The model under review builds one solid part; all positions refer to its coordinate system, in mm. A direction names the side the tool comes from. Round coordinates to 2 decimals unless told otherwise and drop trailing zeros. Loops run counter-clockwise (first coordinate to the right, second up) from the corner with the lowest first, then second, coordinate; pieces in that order, holes last. Notation, with made-up numbers: (31, 38) -> (65, 38) arc R31 ccw to (65, 70) -> close; hole circle Ø10 at (-33.75, -16.75). An arc over 180 degrees is marked (long way). Use a Markdown table: item, result. Add a question column.
1) For faces 4 (the cylindrical face through (1.449, 81.022, 3.219)), 5 (the flat face through (79.375, 41, 5)), list the 3-axis set-ups (+Z, -Z, +X, -X, +Y, -Y) from which the entire face can be reached by the end or side of a thin tool; tool diameter is ignored.
2) Mouldability with a two-part tool opening along X and no side actions: class faces 1 (the flat face through (41, 3.175, 5)), 2 (the flat face through (41, 42, 0)), 3 (the flat face through (0, 41, 3)) as released by +X, released by -X, zero draft, split by the parting line, or undercut.
3) Wall thickness on probe 1 along Y at (x, z) = (6, 5.5) (3 decimals); probe 2 along Z at (x, y) = (64, 55.5) (3 decimals): over which ranges is each line inside the solid? List them lowest first.
4) Consider section B-B on y = 30. Give the boundary of the cut face in (x, z) (3 decimals).
5) Consider section A-A on z = 4.75. Give the boundary of the cut face in (x, y) (3 decimals).
from build123d import *

# Parameters (mm, degrees)
F0_W     = 82.55
F0_H     = 82.55
F1_DEPTH = 6.35
F2_W     = 76.2
F2_H     = 76.2
F3_DEPTH = 3.175
F4_R     = 5.08
F5_R     = 2.54


with BuildPart() as f1:
    # F0 (on Top) → F1 (new body)
    with BuildSketch(Plane.XY):
        with Locations((41.275, 41.275)):
            Rectangle(F0_W, F0_H)
    extrude(amount=F1_DEPTH)

    # F2 (on face) → F3 (cut)
    with BuildSketch(Plane.XY.offset(6.35)):
        with Locations((41.275, 41.275)):
            Rectangle(F2_W, F2_H)
    extrude(amount=-F3_DEPTH, mode=Mode.SUBTRACT)

    # F4
    f4_edges = [f1.edges().sort_by_distance(p)[0] for p in [
        (0, 0, 3.175),
        (82.55, 0, 3.175),
        (82.55, 82.55, 3.175),
        (0, 82.55, 3.175),
    ]]
    fillet(f4_edges, radius=F4_R)

    # F5
    f5_edges = [f1.edges().sort_by_distance(p)[0] for p in [
        (79.375, 3.175, 4.7625),
        (3.175, 3.175, 4.7625),
        (3.175, 79.375, 4.7625),
        (79.375, 79.375, 4.7625),
    ]]
    fillet(f5_edges, radius=F5_R)


solid = f1.part
Result set:
| question | item | result |
|---|---|---|
| 1 | face 4 | +Z, -Z, -X, +Y |
| 1 | face 5 | +Z |
| 2 | face 1 | undercut |
| 2 | face 2 | zero draft |
| 2 | face 3 | released by -X |
| 3 | probe 1 | 0 to 3.175, 79.375 to 82.55 |
| 3 | probe 2 | 0 to 3.175 |
| 4 | outline | (0, 0) -> (82.55, 0) -> (82.55, 6.35) -> (79.375, 6.35) -> (79.375, 3.175) -> (3.175, 3.175) -> (3.175, 6.35) -> (0, 6.35) -> close |
| 5 | outline | (0, 5.08) arc R5.08 ccw to (5.08, 0) -> (77.47, 0) arc R5.08 ccw to (82.55, 5.08) -> (82.55, 77.47) arc R5.08 ccw to (77.47, 82.55) -> (5.08, 82.55) arc R5.08 ccw to (0, 77.47) -> close; hole (3.175, 5.715) arc R2.54 ccw to (5.715, 3.175) -> (76.835, 3.175) arc R2.54 ccw to (79.375, 5.715) -> (79.375, 76.835) arc R2.54 ccw to (76.835, 79.375) -> (5.715, 79.375) arc R2.54 ccw to (3.175, 76.835) -> close |
